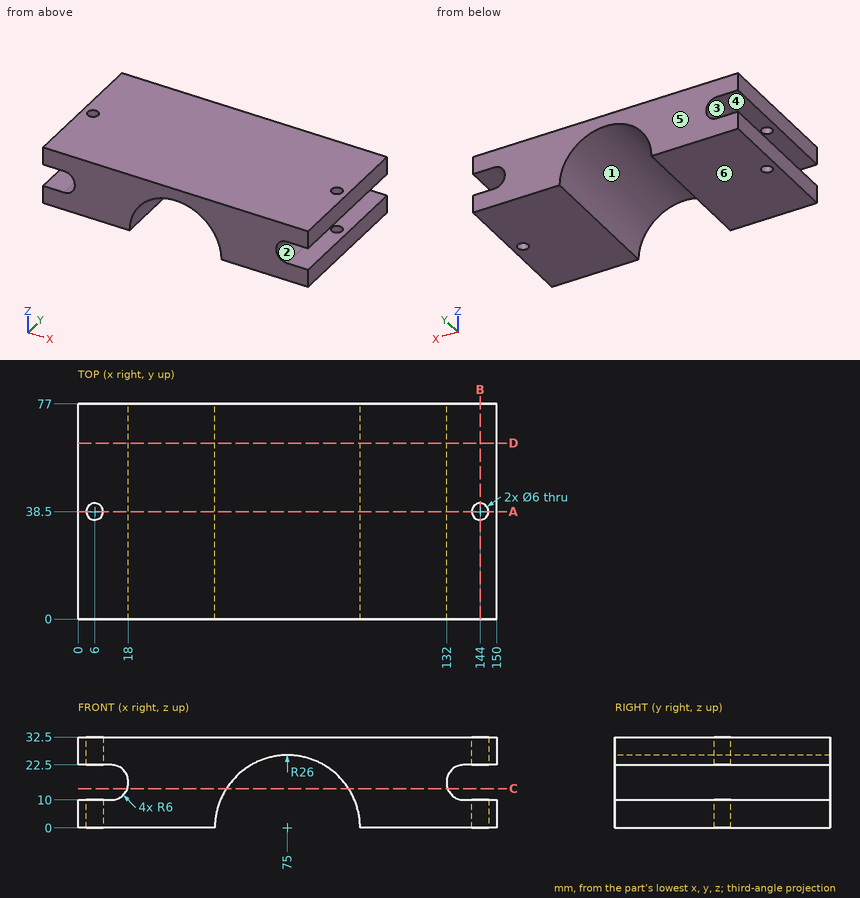
Drawing for the job (mm, zero at the part's lowest x, y, z). A direction names the side the tool comes from. Give positions to 0.01 mm unless a question says otherwise; leave off trailing zeros. Loops run counter-clockwise (first coordinate to the right, second up) from the corner with the lowest first, then second, coordinate; pieces in that order, holes last. Notation, with made-up numbers: M 38,8.5 L 71,8.5 A34 ccw 71,43.5 Z; hole C 61.25,-17 d10. An arc over 180 degrees is marked long. One line per question, with ' | ' between items. Start each with the question number.
1. Saw through at C-C on z = 14. Give the cut face in (x, y).
2. Probe L1, parallel to Y at x = 6, z = 2; L2, parallel to X at y = 55.5, z = 12; L3, parallel to X at y = 45, z = 22. List the from-to ranges inside material, lowest first. Write a range as from..to.
3. Flat gauge pins, fed straight in: pin 1 (1 mm diameter, centred on y = 40.5, z = 13, fed in from +X); pin 2 (6 mm diameter, centred on x = 121.5, y = 10.5, fed in from -Z). Where does each tip first touch, or does it go through?
4. Saw through at B-B on x = 144. Give the cut face in (y, z), plus the area to 3 significant figures.
5. Two-plate mould, pull along Z, no slides. Class the marked faces 4, 5 and 6: pulls with the +Z half, pulls with the -Z half, needs draft (parallel to the pull), parting line crosses it, or undercut.
6. Saw through at A-A on y = 38.5. State how many separate pieces and enclosed holes the cut face has, plus the area to 3 significant figures.
7. Saw through at D-D on y = 63. Give the cut face in (x, z).
8. 3-axis set-ups, long thin cutter, end or side, ignore diameter. For the marked faces 1, 2 and 3: which of +Z, -Z, +X, -X, +Y, -Y reach the whole face in a straight line?
Result sheet:
1) outline: M 17.66,0 L 53.09,0 L 53.09,77 L 17.66,77 Z; M 96.91,0 L 132.34,0 L 132.34,77 L 96.91,77 Z
2) L1: y = 0..35.5, 41.5..77 | L2: x = 16.47..51.93, 98.07..133.53 | L3: x = 14.4..61.14, 88.86..135.6
3) pin 1: stops at x = 133.13 | pin 2: stops at z = 0
4) outline: M 0,0 L 35.5,0 L 35.5,10 L 0,10 Z; M 0,22.5 L 35.5,22.5 L 35.5,32.5 L 0,32.5 Z; M 41.5,0 L 77,0 L 77,10 L 41.5,10 Z; M 41.5,22.5 L 77,22.5 L 77,32.5 L 41.5,32.5 Z | area: 1,420 mm^2
5) face 4: undercut | face 5: needs draft | face 6: pulls with the -Z half
6) separate pieces: 5 | enclosed holes: 0 | area: 3,150 mm^2
7) outline: M 0,0 L 49,0 A26 cw 101,0 L 150,0 L 150,10 L 138,10 A6 cw 132,16 L 132,16.5 A6 cw 138,22.5 L 150,22.5 L 150,32.5 L 0,32.5 L 0,22.5 L 12,22.5 A6 cw 18,16.5 L 18,16 A6 cw 12,10 L 0,10 Z
8) face 1: -Z, +Y, -Y | face 2: +X, +Y, -Y | face 3: -X, +Y, -Y
